from build123d import *

# Parameters (mm, degrees)
SKETCH_1_W          = 19.7
SKETCH_1_H          = 25.65
SKETCH_1_R          = 3.25
SKETCH_1_R_2        = 1
EXTRUDE_1_DEPTH     = 3
SKETCH_1_3_W        = 3.85
SKETCH_1_3_H        = 8.3
EXTRUDE_2_DEPTH     = 8
FILLET_1_R          = 2
CHAMFER_1_SIZE      = 2.9
FILLET_2_R          = 1
EXTRUDE_START       = 3
EXTRUDE_4_DEPTH     = 1.4
FILLET_3_R          = 1
CUT_EXTRUDE_START   = 1.4
SKETCH_1_5_R        = 1
CUT_EXTRUDE_1_DEPTH = 1.6


with BuildPart() as part:
    # Эскиз1 → Бобышка-Вытянуть1 (new body)
    with BuildSketch(Plane.XY):
        with Locations((8.965987089, 2.175)):
            Rectangle(SKETCH_1_W, SKETCH_1_H)
        with Locations((8.965987089, 0)):
            Circle(SKETCH_1_R, mode=Mode.SUBTRACT)
        with Locations((4.115987089, 9.774393406)):
            Circle(SKETCH_1_R_2, mode=Mode.SUBTRACT)
        with Locations((13.815987089, 9.774393406)):
            Circle(SKETCH_1_R_2, mode=Mode.SUBTRACT)
    extrude(amount=EXTRUDE_1_DEPTH)

    # Эскиз1<3> → Бобышка-Вытянуть2 (add)
    with BuildSketch(Plane.XY):
        with Locations((1.040987089, 0)):
            Rectangle(SKETCH_1_3_W, SKETCH_1_3_H)
        with Locations((16.890987089, 0)):
            Rectangle(SKETCH_1_3_W, SKETCH_1_3_H)
    extrude(amount=EXTRUDE_2_DEPTH)

    # Скругление1
    fillet_1_edges = [part.edges().sort_by_distance(p)[0] for p in [
        (-0.884012911, -10.65, 1.5),
        (-0.884012911, 15, 1.5),
        (18.815987089, 15, 1.5),
        (18.815987089, -10.65, 1.5),
    ]]
    fillet(fillet_1_edges, radius=FILLET_1_R)

    # Фаска1
    chamfer_1_edges = [part.edges().sort_by_distance(p)[0] for p in [
        (5.715987089, 0, 0),
    ]]
    chamfer(chamfer_1_edges, length=CHAMFER_1_SIZE)

    # Скругление2
    fillet_2_edges = [part.edges().sort_by_distance(p)[0] for p in [
        (-0.884012911, 4.15, 5.5),
        (-0.884012911, -4.15, 5.5),
        (18.815987089, -4.15, 5.5),
        (18.815987089, 4.15, 5.5),
    ]]
    fillet(fillet_2_edges, radius=FILLET_2_R)

    # Эскиз1<4> → Бобышка-Вытянуть4 (add)
    with BuildSketch(Plane.XY.offset(EXTRUDE_START)):
        with BuildLine():
            Line((2.965987089, 0), (2.965987089, -4.15))
            Line((2.965987089, -4.15), (14.965987089, -4.15))
            Line((14.965987089, -4.15), (14.965987089, 0))
            Line((14.965987089, 0), (12.215987089, 0))
            ThreePointArc((12.215987089, 0), (8.965987089, -3.25), (5.715987089, 0))
            Line((5.715987089, 0), (2.965987089, 0))
        make_face()
        with BuildLine():
            Line((14.965987089, 4.15), (2.965987089, 4.15))
            Line((2.965987089, 4.15), (2.965987089, 0))
            Line((2.965987089, 0), (5.715987089, 0))
            ThreePointArc((5.715987089, 0), (8.965987089, 3.25), (12.215987089, 0))
            Line((12.215987089, 0), (14.965987089, 0))
            Line((14.965987089, 0), (14.965987089, 4.15))
        make_face()
    extrude(amount=EXTRUDE_4_DEPTH)

    # Скругление3
    fillet_3_edges = [part.edges().sort_by_distance(p)[0] for p in [
        (2.965987089, -4.15, 6.2),
        (2.965987089, 4.15, 6.2),
        (14.965987089, -4.15, 6.2),
        (14.965987089, 4.15, 6.2),
    ]]
    fillet(fillet_3_edges, radius=FILLET_3_R)

    # Эскиз1<5> → Вырез-Вытянуть1 (cut)
    with BuildSketch(Plane.XY.offset(CUT_EXTRUDE_START)):
        Polygon((6.265987089, 8.533090327), (6.265987089, 11.015696485), (4.115987089, 12.256999563), (1.965987089, 11.015696485), (1.965987089, 8.533090327), (4.115987089, 7.291787248), align=None)
        with Locations((4.115987089, 9.774393406)):
            Circle(SKETCH_1_5_R, mode=Mode.SUBTRACT)
        Polygon((15.965987089, 8.533090327), (15.965987089, 11.015696485), (13.815987089, 12.256999563), (11.665987089, 11.015696485), (11.665987089, 8.533090327), (13.815987089, 7.291787248), align=None)
        with Locations((13.815987089, 9.774393406)):
            Circle(SKETCH_1_5_R, mode=Mode.SUBTRACT)
    extrude(amount=CUT_EXTRUDE_1_DEPTH, mode=Mode.SUBTRACT)


solid = part.part
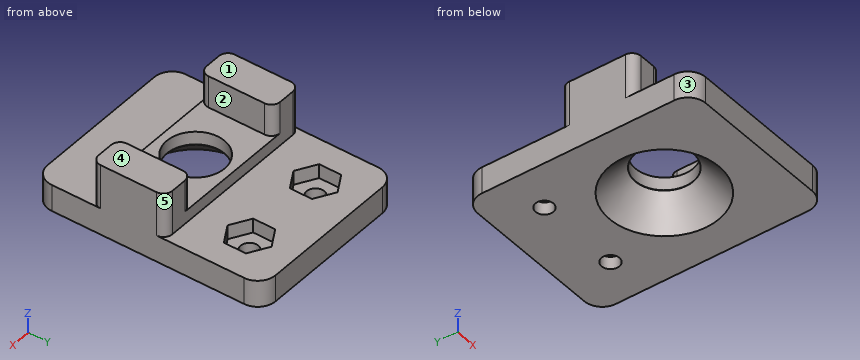
Work out the finished part from the listing and answer in its coordinate system (mm). Face numbers are marked on the shaded views. A direction names the side the tool comes from. Round coordinates to 2 decimals unless told otherwise and drop trailing zeros. Write each loop counter-clockwise with the first axis right and the second up, starting at its lowest first coordinate (ties: lowest second). Pieces come first, ordered by that corner, then holes.
1) A cutting plane is placed at B-B (z = 6). Give the vertices of the cut face in (x, y), plus the area to 3 significant figures.
2) A cutting plane is placed at A-A (y = 0). Give the vertices of the cut face in (x, z).
3) A cutting plane is placed at C-C (x = 0.5). Give the vertices of the cut face in (y, z), plus the area to 3 significant figures.
4) The mould has two halves that part along X. Classify the marked faces 1, 2 and 3: pulls with the +X half, pulls with the -X half, needs draft (parallel to the pull), parting line crosses it, or undercut.
5) Straight lines are drawn through the part: line 1 (X direction, y = -2.5, z = 6.75); line 2 (Y direction, x = 6, z = 2.25); line 3 (X direction, y = 10, z = 1.25). For each, find the intervals that lie inside material, in ascending order.
6) A tool of negligible diameter and unlimited length cuts with its end or side. For the marked faces 4 and 5, from which of +Z, -Z, +X, -X, +Y, -Y can it reach the whole face along a straight path? Write none if from no direction.
7) Given pin 1 Ø1.5 at (x, z) = (12.5, 5) entering from -Y; pin 2 Ø1.3 at (x, y) = (13.5, 10) entering from +Z; pin 3 Ø7.5 at (x, y) = (8.97, 0) entering from -Z, each flat-ended and moving along its own axis, determine where each tip first touches the part or whether it passes through.
Completed:
1. outline: (-0.88, -3.15) arc R1 ccw to (0.12, -4.15) - (1.97, -4.15) arc R1 ccw to (2.97, -3.15) - (2.97, 3.15) arc R1 ccw to (1.97, 4.15) - (0.12, 4.15) arc R1 ccw to (-0.88, 3.15) - close; (14.97, -3.15) arc R1 ccw to (15.97, -4.15) - (17.82, -4.15) arc R1 ccw to (18.82, -3.15) - (18.82, 3.15) arc R1 ccw to (17.82, 4.15) - (15.97, 4.15) arc R1 ccw to (14.97, 3.15) - close
1. area: 62.2 mm2
2. outline: (-0.88, 0) - (2.82, 0) - (5.72, 2.9) - (5.72, 4.4) - (2.97, 4.4) - (2.97, 8) - (-0.88, 8) - close; (12.22, 2.9) - (15.12, 0) - (18.82, 0) - (18.82, 8) - (14.97, 8) - (14.97, 4.4) - (12.22, 4.4) - close
3. outline: (-10.55, 0) - (14.9, 0) - (14.9, 3) - (4.15, 3) - (4.15, 8) - (-4.15, 8) - (-4.15, 3) - (-10.55, 3) - close
3. area: 118 mm2
4. face 1: needs draft
4. face 2: undercut
4. face 3: pulls with the -X half
5. line 1: x = -0.88 to 2.97, 14.97 to 18.82
5. line 2: y = -10.65 to -2.53, 2.53 to 8.38, 11.17 to 15
5. line 3: x = -0.88 to 3.14, 5.09 to 12.84, 14.79 to 18.82
6. face 4: +Z, +X, -X, +Y, -Y
6. face 5: +Z, +X, +Y
7. pin 1: stops at y = -4.15
7. pin 2: stops at z = 1.4
7. pin 3: stops at z = 2.4
